Source: CAD feature listing. Evaluate the final solid. Frame: model axes, mm. Face numbers are marked on the shaded views. A direction names the side the tool comes from. Give positions to 0.01 mm unless a question says otherwise; leave off trailing zeros. Write each loop counter-clockwise with the first axis right and the second up, starting at its lowest first coordinate (ties: lowest second). Pieces come first, ordered by that corner, then holes.
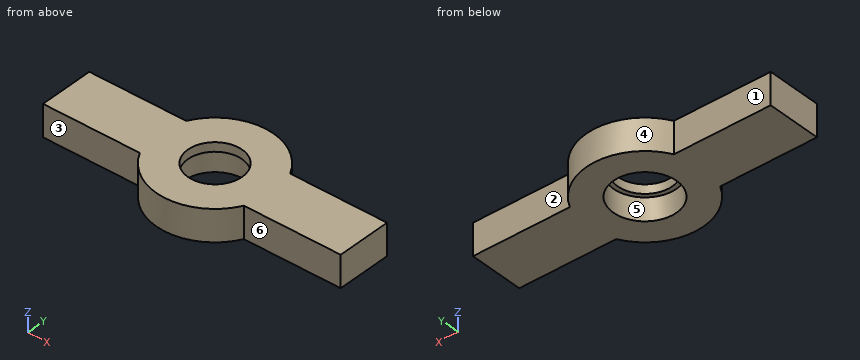
```python
from build123d import *

# Parameters (mm, degrees)
RESSALTO_EXTRUS_O1_DEPTH = 35
ESBO_O2_R                = 35
CORTE_EXTRUS_O1_DEPTH    = 25
ESBO_O3_R                = 30
CORTE_EXTRUS_O2_DEPTH    = 477.313972081


with BuildPart() as part:
    # Esboço1 → Ressalto-extrusão1 (new body)
    with BuildSketch(Plane.XY):
        with BuildLine():
            Line((-257.662812973, -210), (-365, -210))
            Line((-365, -210), (-365, -270))
            Line((-365, -270), (-257.662812973, -270))
            ThreePointArc((-257.662812973, -270), (-200, -305), (-142.337187027, -270))
            Line((-142.337187027, -270), (-35, -270))
            Line((-35, -270), (-35, -210))
            Line((-35, -210), (-142.337187027, -210))
            ThreePointArc((-142.337187027, -210), (-200, -175), (-257.662812973, -210))
        make_face()
    extrude(amount=-RESSALTO_EXTRUS_O1_DEPTH)

    # Esboço2 → Corte-extrusão1 (cut)
    with BuildSketch(Plane(origin=(0, 0, -35), x_dir=(-1, 0, 0), z_dir=(0, 0, -1))):
        with Locations((200, -240)):
            Circle(ESBO_O2_R)
    extrude(amount=-CORTE_EXTRUS_O1_DEPTH, mode=Mode.SUBTRACT)

    # Esboço3 → Corte-extrusão2 (cut, through all)
    with BuildSketch(Plane(origin=(0, 0, -10), x_dir=(-1, 0, 0), z_dir=(0, 0, -1))):
        with Locations((200, -240)):
            Circle(ESBO_O3_R)
    extrude(amount=-CORTE_EXTRUS_O2_DEPTH, mode=Mode.SUBTRACT)


solid = part.part
```
1. Pull-direction query (Y, two-part tool) for the marked faces 4, 5 and 6; classes: pulls with the +Y half, pulls with the -Y half, needs draft (parallel to the pull), parting line crosses it, or undercut.
2. Access query for the marked faces 1, 2 and 3. Directions: +Z, -Z, +X, -X, +Y, -Y. A direction counts if a zero-diameter tool reaches every point of the face in a straight line with its end or side. Return the directions, or none.
3. Section query C-C (z = -6). Return loops of the section in (x, y), plus the area to 3 significant figures.
4. Section query B-B (y = -240). Return loops of the section in (x, z), plus the area to 3 significant figures.
5. Section query A-A (x = -200). Return loops of the section in (y, z), plus the area to 3 significant figures.
6. Pin query (flat end, axial travel): P1, Ø5, axis at y = -205, z = -14, coming from the +X side; P2, Ø6, axis at x = -264, y = -241, coming from the +Z side; P3, Ø5, axis at x = -329, z = -27.5, coming from the +Y side; P4, Ø1, axis at x = -127, z = -8.5, coming from the -Y side. Return the tip coordinate at first contact, or that it passes through.
7. Section query D-D (z = -28.5). Return loops of the section in (x, y), plus the area to 3 significant figures.
8. Line query: probe 1 along Y at (x, z) = (-200, -3); probe 2 along Y at (x, z) = (-322, -25); probe 3 along Y at (x, z) = (-200, -24.5). Output: solid intervals per line, ascending.
The answers:
1. face 4: pulls with the +Y half
1. face 5: undercut
1. face 6: pulls with the -Y half
2. face 1: +Z, -Z, -X, +Y
2. face 2: +Z, -Z, +X, +Y
2. face 3: +Z, -Z, -X, -Y
3. outline: (-365, -270) - (-257.66, -270) arc R65 ccw to (-142.34, -270) - (-35, -270) - (-35, -210) - (-142.34, -210) arc R65 ccw to (-257.66, -210) - (-365, -210) - close; hole circle Ø60 at (-200, -240)
3. area: 22,700 mm2
4. outline: (-365, -35) - (-235, -35) - (-235, -10) - (-230, -10) - (-230, 0) - (-365, 0) - close; (-170, -10) - (-165, -10) - (-165, -35) - (-35, -35) - (-35, 0) - (-170, 0) - close
4. area: 9,200 mm2
5. outline: (-305, -35) - (-275, -35) - (-275, -10) - (-270, -10) - (-270, 0) - (-305, 0) - close; (-210, -10) - (-205, -10) - (-205, -35) - (-175, -35) - (-175, 0) - (-210, 0) - close
5. area: 2,200 mm2
6. P1: stops at x = -143.71
6. P2: stops at z = 0
6. P3: stops at y = -210
6. P4: stops at y = -270
7. outline: (-365, -270) - (-257.66, -270) arc R65 ccw to (-142.34, -270) - (-35, -270) - (-35, -210) - (-142.34, -210) arc R65 ccw to (-257.66, -210) - (-365, -210) - close; hole circle Ø70 at (-200, -240)
7. area: 21,700 mm2
8. probe 1: y = -305 to -270, -210 to -175
8. probe 2: y = -270 to -210
8. probe 3: y = -305 to -275, -205 to -175
